Read the model definition and answer for the solid it produces. Units are mm, in the model's axes. A direction names the side the tool comes from. Give positions to 0.01 mm unless a question says otherwise; leave off trailing zeros. Order: outer loops, then holes, each group sorted by start corner. A loop starts at its lowest first (then second) coordinate and runs counter-clockwise, first axis right, second up. Notation, with made-up numbers: M -16,-33.5 L -8,-33.5 A16 cw -8,-21.5 Z; hole C 7.25,6 d11. An arc over 180 degrees is marked long. One line per item, written item: value. Start each with the question number.
from build123d import *

# Parameters (mm, degrees)
F0_R     = 46.355
F1_DEPTH = 6.35
F2_R     = 24.892
F2_R_2   = 14.732
F3_DEPTH = 12.7
F4_W     = 1.27
F4_H     = 2.794
F6_R     = 0.254


with BuildPart() as f1:
    # F0 (on Top) → F1 (new body)
    with BuildSketch(Plane.XY):
        Circle(F0_R)
    extrude(amount=F1_DEPTH)

    # F2 (on face) → F3 (join)
    with BuildSketch(Plane.XY.offset(6.35)):
        Circle(F2_R)
        Circle(F2_R_2, mode=Mode.SUBTRACT)
    extrude(amount=F3_DEPTH)

    # F4 (on Front) → F5 (revolve, cut)
    with BuildSketch(Plane.XZ):
        with Locations((24.257, 10.287)):
            Rectangle(F4_W, F4_H)
    revolve(axis=Axis((0, 0, 4.445), (0, 0, 1)), mode=Mode.SUBTRACT)

    # F6
    f6_edges = [f1.edges().sort_by_distance(p)[0] for p in [
        (-23.622, 0, 11.684),
        (-23.622, 0, 8.89),
    ]]
    fillet(f6_edges, radius=F6_R)


solid = f1.part
Q1. Find section D-D, the plane y = 39.5. Give the vertices of the cut face in (x, z), then the cut area to 3 significant figures.
Q2. Find section C-C, the plane z = 3. Give the vertices of the cut face in (x, y) (3 decimals), then the cut area to 3 significant figures.
Q3. Each of these flat-tipped pins is pushed along its axis until it touches: pin 1 (3 mm diameter, centred on y = 24.5, z = 4.5, fed in from +X); pin 2 (4 mm diameter, centred on x = -8, z = 5.5, fed in from -Y); pin 3 (10 mm diameter, centred on x = 22.5, z = 7.5, fed in from -Y). Where does it stop, or does it pass through?
Q4. Consider probe 1 along Y at (x, z) = (0, 14.75); probe 2 along Z at (x, y) = (-6, 24); probe 3 along Z at (x, y) = (16, 29.5). Determine where each line is inside the solid, lowest interval first.
Q5. A tool of negligible diameter and unlimited length cuts with its end or side. For faces 4 (the cylindrical face through (-5.4, -24.3, 15.3)), 5 (the cylindrical face through (42.8, -17.8, 3.1)), 6 (the flat face through (-2, -24, 11.684)), from which of +Z, -Z, +X, -X, +Y, -Y can it reach the whole face along a straight path? Write none if from no direction.
Q6. Find section A-A, the plane x = 0. Give the vertices of the cut face in (y, z) (3 decimals), then the cut area to 3 significant figures.
Q7. Determine the mould class of faces 1 (the flat face through (-1, 1, 0)), 2 (the flat face through (20, -20, 6.35)), 3 (the cylindrical face through (-18.75, -14.37, 10.3)) for opening direction Z: released by +Z, released by -Z, zero draft, split by the parting line, or undercut.
Evaluation:
1. outline: M -24.26,0 L 24.26,0 L 24.26,6.35 L -24.26,6.35 Z
1. area: 308 mm2
2. outline: C 0,0 d92.71
2. area: 6,750 mm2
3. pin 1: x = 40.25
3. pin 2: y = -45.97
3. pin 3: y = -42.87
4. probe 1: -24.89 to -14.73, 14.73 to 24.89
4. probe 2: 0 to 8.89, 11.68 to 19.05
4. probe 3: 0 to 6.35
5. face 4: +Z
5. face 5: +Z, -Z
5. face 6: none
6. outline: M -46.355,0 L 46.355,0 L 46.355,6.35 L 24.892,6.35 L 24.892,8.89 L 23.876,8.89 A0.254 cw 23.622,9.144 L 23.622,11.43 A0.254 cw 23.876,11.684 L 24.892,11.684 L 24.892,19.05 L 14.732,19.05 L 14.732,6.35 L -14.732,6.35 L -14.732,19.05 L -24.892,19.05 L -24.892,11.684 L -23.876,11.684 A0.254 cw -23.622,11.43 L -23.622,9.144 A0.254 cw -23.876,8.89 L -24.892,8.89 L -24.892,6.35 L -46.355,6.35 Z
6. area: 840 mm2
7. face 1: released by -Z
7. face 2: released by +Z
7. face 3: undercut
